Study the drawing (mm; zero at the part's minimum x, y, z) and answer. A direction names the side the tool comes from. Coordinates: 2 decimals unless noted, no trailing zeros. Order: outer loops, then holes, each group sorted by start corner. A loop starts at its lowest first (then second) coordinate and runs counter-clockwise, first axis right, second up.
1. The part is cut by section A-A, the plane x = 32. Give the vertices of the cut face in (y, z).
2. Flat-ended cylindrical pins translate along their axes: pin 1 Ø3 at (y, z) = (11.5, 28) entering from -X; pin 2 Ø1.5 at (y, z) = (6.5, 71) entering from +X. Find the tip coordinate at first contact, or state that the pin passes through.
3. The part is cut by section D-D, the plane z = 59. Give the vertices of the cut face in (x, y).
4. Find the intervals of material crossed by probe 1 along Z at (x, y) = (36, 24.5); probe 2 along X at (y, z) = (10, 10.5), in increasing order.
5. The part is cut by section C-C, the plane x = 17. Give the vertices of the cut face in (y, z).
6. The part is cut by section B-B, the plane y = 21. Count the separate pieces of the cut face and the enclosed holes in it, then the cut area to 3 significant figures.
7. A tool of negligible diameter and unlimited length cuts with its end or side. For the marked faces 5 and 6, from which of +Z, -Z, +X, -X, +Y, -Y can it reach the whole face along a straight path? Write none if from no direction.
8. Determine the mould class of the marked faces 1, 2, 3 and 4 for opening direction Z: +Z half, -Z half, draft (parallel to the pull), parting line (faces both ways), or undercut.
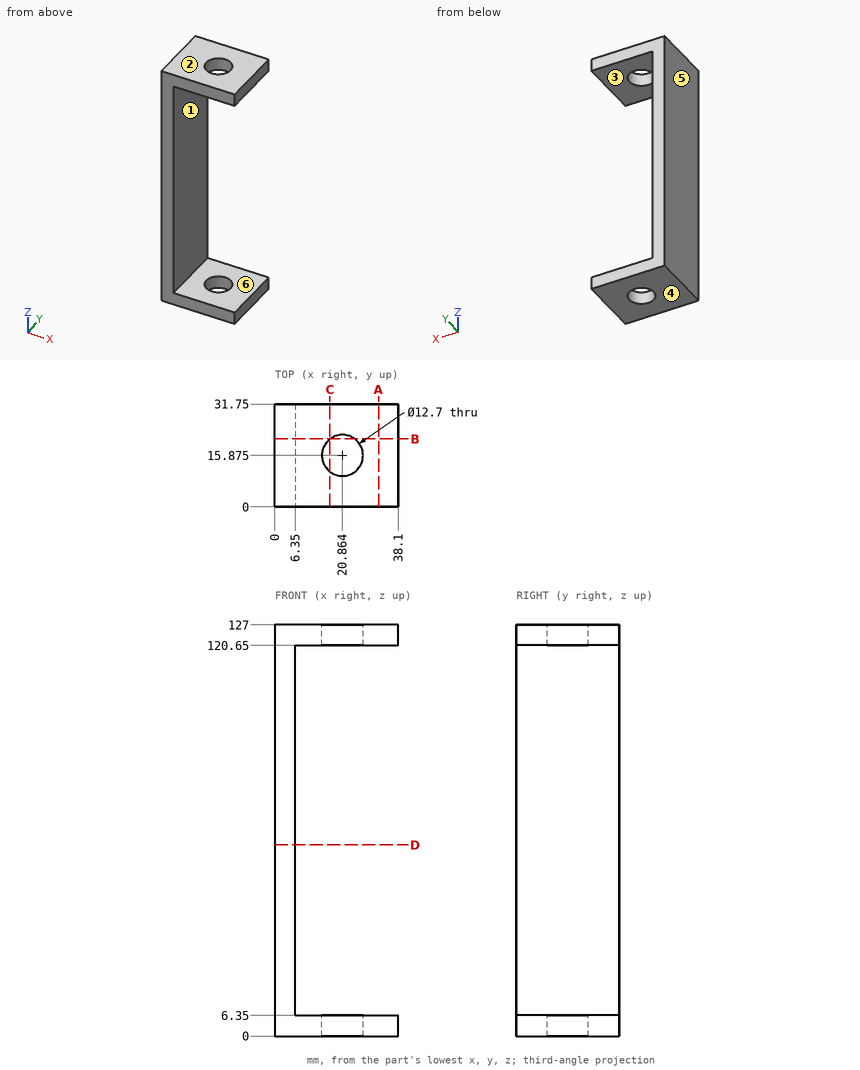
Geometry says:
1. outline: (0, 0) - (31.75, 0) - (31.75, 6.35) - (0, 6.35) - close; (0, 120.65) - (31.75, 120.65) - (31.75, 127) - (0, 127) - close
2. pin 1: stops at x = 0
2. pin 2: stops at x = 6.35
3. outline: (0, 0) - (6.35, 0) - (6.35, 31.75) - (0, 31.75) - close
4. probe 1: z = 0 to 6.35, 120.65 to 127
4. probe 2: x = 0 to 6.35
5. outline: (0, 0) - (10.84, 0) - (10.84, 6.35) - (0, 6.35) - close; (0, 120.65) - (10.84, 120.65) - (10.84, 127) - (0, 127) - close; (20.91, 0) - (31.75, 0) - (31.75, 6.35) - (20.91, 6.35) - close; (20.91, 120.65) - (31.75, 120.65) - (31.75, 127) - (20.91, 127) - close
6. separate pieces: 3
6. enclosed holes: 0
6. area: 1,110 mm2
7. face 5: +Z, -Z, -X, +Y, -Y
7. face 6: +X, +Y, -Y
8. face 1: undercut
8. face 2: +Z half
8. face 3: undercut
8. face 4: -Z half
